Part model, mm, in its own coordinate system. Coordinates: 2 decimals unless noted, no trailing zeros. Loops run counter-clockwise (first coordinate to the right, second up) from the corner with the lowest first, then second, coordinate; pieces in that order, holes last. Notation, with made-up numbers: (81, -10) - (95, -10) arc R20 ccw to (95, 1) - close; hole circle Ø4 at (-18.5, 27.5). An arc over 180 degrees is marked (long way). Use a Markdown table: item, result. Add a question column.
1) Probe probe 1 along X at (y, z) = (2.55, 103); probe 2 along Z at (x, y) = (-29, 2.05); probe 3 along X at (y, z) = (2.7, -142). List the from-to ranges inside material, lowest first. Write a range as [from, to].
2) Drop a flat-ended pin along its axis: P1, Ø1.5, axis at y = 2, z = 100, coming from the -X side (3 decimals). Give the stop position or say it passes through.
3) Band-saw the part on C-C (x = -131.5). Give the cut face in (y, z), plus the area to 3 significant figures.
4) Band-saw the part on B-B (z = -9). Give the cut face in (x, y).
5) Band-saw the part on A-A (y = 1.7). Give the cut face in (x, z).
6) Pull direction X, two halves, no side cores. Call faces 1 (the face through (-28.141, 1.479, 107.377)), 2 (the face through (-76, 3, -53)), 3 (the face through (-140.924, 1.479, 51.42)): +X half, -X half, draft (parallel to the pull), parting line (faces both ways), or undercut.
Autodesk Inventor part; units mm, degrees
ref_plane "YZ Plane" through (0, 0, 0) normal (1, 0, 0) x (0, 1, 0)
ref_plane "XZ Plane" through (0, 0, 0) normal (0, 1, 0) x (-1, 0, 0)
ref_plane "XY Plane" through (0, 0, 0) normal (0, 0, 1) x (1, 0, 0)
sketch "スケッチ1" plane through (0, 0, 0) normal (0, 1, 0) x (-1, 0, 0)
  line L0 (0, 254.5) -> (0, -254.5)
  line L1 (0, -254.5) -> (200, -254.5)
  line L2 (200, -254.5) -> (200, -145.5)
  line L3 (200, -145.5) -> (80, 254.5)
  line L4 (80, 254.5) -> (0, 254.5)
  point P0 (0, 0)
  point P1 (0, 0)
  dimension "d0" = 509
  dimension "d1" = 200
  dimension "d2" = 109
  dimension "d3" = 80
extrude "押し出し1" add sketch "スケッチ1" along normal blind 3
sketch "スケッチ2" plane through (0, 0, 0) normal (0, -1, 0) x (1, 0, 0)
  circle A0 centre (-35.142, 214.391) radius 4.25
  circle A1 centre (-30.426, 103.793) radius 4.25
  line L0 (-65, 84.5) -> (-50, 84.5)
  line L1 (-50, 84.5) -> (-50, 114.5)
  line L2 (-50, 114.5) -> (-65, 114.5)
  line L3 (-65, 114.5) -> (-65, 84.5)
  line L4 (-80, 254.5) -> (0, 254.5)
  line L5 (0, 254.5) -> (0, -254.5)
  point P0 (0, 0)
  dimension "d6" = 15
  dimension "d7" = 30
  dimension "d8" = 8.5
  dimension "d9" = 8.5
  dimension "d10" = 40.109
  dimension "d11" = 35.142
  dimension "d12" = 150.707
  dimension "d13" = 30.426
  dimension "d14" = 140
  dimension "d15" = 50
extrude "押し出し2" cut sketch "スケッチ2" against normal blind 3
fillet "フィレット1" radius 1 9 edges at (-80, 1.5, 254.5) (0, 1.5, 254.5) (-200, 1.5, -145.5) (-200, 1.5, -254.5) (0, 1.5, -254.5) (-50, 1.5, 84.5) (-50, 1.5, 114.5) (-65, 1.5, 114.5) (-65, 1.5, 84.5)
Answer block:
| question | item | result |
|---|---|---|
| 1 | probe 1 | [-125.45, -65], [-50, -34.6], [-26.25, 0] |
| 1 | probe 2 | [-254.5, 99.79], [107.8, 254.5] |
| 1 | probe 3 | [-198.95, 0] |
| 2 | P1 | x = -126.575 |
| 3 | outline | (0, -254.5) - (3, -254.5) - (3, 82.83) - (0, 82.83) - close |
| 3 | area | 1,010 mm2 |
| 4 | outline | (-159.05, 0) - (0, 0) - (0, 3) - (-159.05, 3) - close |
| 5 | outline | (-200, -253.5) arc R1 ccw to (-199, -254.5) - (-1, -254.5) arc R1 ccw to (0, -253.5) - (0, 253.5) arc R1 ccw to (-1, 254.5) - (-79.26, 254.5) arc R1 ccw to (-80.21, 253.79) - (-199.96, -145.36) arc R1 ccw to (-200, -145.65) - close; hole (-65, 85.5) arc R1 ccw to (-64, 84.5) - (-51, 84.5) arc R1 ccw to (-50, 85.5) - (-50, 113.5) arc R1 ccw to (-51, 114.5) - (-64, 114.5) arc R1 ccw to (-65, 113.5) - close; hole circle Ø8.5 at (-35.14, 214.39); hole circle Ø8.5 at (-30.43, 103.79) |
| 6 | face 1 | undercut |
| 6 | face 2 | draft |
| 6 | face 3 | -X half |
